```python
from build123d import *

# Parameters (mm, degrees)
SKETCH1_R           = 62.5
SKETCH1_R_2         = 1.75
SKETCH1_R_3         = 19.5
BOSS_EXTRUDE1_DEPTH = 2


with BuildPart() as part:
    # Sketch1 → Boss-Extrude1 (new body)
    with BuildSketch(Plane(origin=(0, 0, 0), x_dir=(1, 0, 0), z_dir=(0, 1, 0))):
        with Locations(Location((0, 0, 0), (0, 0, 270))):
            Circle(SKETCH1_R)
        with Locations(Location((6.153691309, -23.5, 0), (0, 0, 270))):
            Circle(SKETCH1_R_2, mode=Mode.SUBTRACT)
        with Locations(Location((-5.846308691, -23.5, 0), (0, 0, 270))):
            Circle(SKETCH1_R_2, mode=Mode.SUBTRACT)
        with Locations(Location((6.153691309, -56.5, 0), (0, 0, 270))):
            Circle(SKETCH1_R_2, mode=Mode.SUBTRACT)
        with Locations(Location((-5.846308691, -56.5, 0), (0, 0, 270))):
            Circle(SKETCH1_R_2, mode=Mode.SUBTRACT)
        with Locations(Location((-46.007280968, 33.313051845, 0), (0, 0, 270))):
            Circle(SKETCH1_R_2, mode=Mode.SUBTRACT)
        with Locations(Location((-23.428442643, 6.420747, 0), (0, 0, 270))):
            Circle(SKETCH1_R_2, mode=Mode.SUBTRACT)
        with Locations(Location((-17.428442643, 16.813051845, 0), (0, 0, 270))):
            Circle(SKETCH1_R_2, mode=Mode.SUBTRACT)
        with Locations(Location((-52.007280968, 22.920747, 0), (0, 0, 270))):
            Circle(SKETCH1_R_2, mode=Mode.SUBTRACT)
        with Locations(Location((51.853589659, 23.186948155, 0), (0, 0, 270))):
            Circle(SKETCH1_R_2, mode=Mode.SUBTRACT)
        with Locations(Location((17.274751335, 17.079253, 0), (0, 0, 270))):
            Circle(SKETCH1_R_2, mode=Mode.SUBTRACT)
        with Locations(Location((23.274751335, 6.686948155, 0), (0, 0, 270))):
            Circle(SKETCH1_R_2, mode=Mode.SUBTRACT)
        with Locations(Location((45.853589659, 33.579253, 0), (0, 0, 270))):
            Circle(SKETCH1_R_2, mode=Mode.SUBTRACT)
        with Locations(Location((0, 0, 0), (0, 0, 270))):
            Circle(SKETCH1_R_3, mode=Mode.SUBTRACT)
        with Locations(Location((0, 30, 0), (0, 0, 270))):
            Circle(SKETCH1_R_2, mode=Mode.SUBTRACT)
        with Locations(Location((25.980762114, -15, 0), (0, 0, 270))):
            Circle(SKETCH1_R_2, mode=Mode.SUBTRACT)
        with Locations(Location((-25.980762114, -15, 0), (0, 0, 270))):
            Circle(SKETCH1_R_2, mode=Mode.SUBTRACT)
    extrude(amount=BOSS_EXTRUDE1_DEPTH)


solid = part.part
```
CAD build for the part. Positions are in the model's coordinates, mm. Coordinates: 2 decimals unless noted, no trailing zeros. Write each loop counter-clockwise with the first axis right and the second up, starting at its lowest first coordinate (ties: lowest second). Pieces come first, ordered by that corner, then holes. Notation, with made-up numbers: (-7, 63) -> (41, 63) arc R26 cw to (41, 95) -> close; hole circle Ø6 at (0, 2). An arc over 180 degrees is marked (long way). Return JSON: item names as keys, results as strings. Group by question number.
Q1. Flat gauge pins, fed straight in: pin 1 (4.5 mm diameter, centred on x = -17.43, z = -16.81, fed in from +Y); pin 2 (1 mm diameter, centred on y = 0.5, z = 39.5, fed in from +X). Where does each tip first touch, or does it go through?
Q2. Cut at C-C, the plane y = 1.35. State how many separate pieces and enclosed holes the cut face has, then the cut area to 3 significant figures.
Q3. Cut at B-B, the plane z = 0. Give the cut face in (x, y), then the cut area to 3 significant figures.
Q4. Drill centre lines: line 1 (X direction, y = 0.2, z = 55); line 2 (X direction, y = 1.2, z = 0); line 3 (X direction, y = 1.2, z = 23.5). Where is each one in solid material? Low to high.
Q5. Pull direction X, two halves, no side cores. Call faces 1 (the face through (2.75, 0.99, -62.44)), 2 (the face through (15, 2, 13)), 3 (the face through (-25.46, 0.99, 16.67)): released by +X, released by -X, zero draft, split by the parting line, or undercut.
Q6. Cut at A-A, the plane x = 0. Give the cut face in (y, z).
Q7. Cut at D-D, the plane z = 15. Give the cut face in (x, y).
Returned:
{
 "1": {"pin 1": "stops at y = 2", "pin 2": "stops at x = 48.84"},
 "2": {"separate pieces": "1", "enclosed holes": "16", "area": "10,900 mm2"},
 "3": {"outline": "(-62.5, 0) -> (-19.5, 0) -> (-19.5, 2) -> (-62.5, 2) -> close; (19.5, 0) -> (62.5, 0) -> (62.5, 2) -> (19.5, 2) -> close", "area": "172 mm2"},
 "4": {"line 1": "x = -29.69 to -6.75, -4.94 to 5.25, 7.06 to 29.69", "line 2": "x = -62.5 to -19.5, 19.5 to 62.5", "line 3": "x = -57.91 to -7.6, -4.1 to 4.4, 7.9 to 57.91"},
 "5": {"face 1": "split by the parting line", "face 2": "zero draft", "face 3": "undercut"},
 "6": {"outline": "(0, -62.5) -> (2, -62.5) -> (2, -31.75) -> (0, -31.75) -> close; (0, -28.25) -> (2, -28.25) -> (2, -19.5) -> (0, -19.5) -> close; (0, 19.5) -> (2, 19.5) -> (2, 62.5) -> (0, 62.5) -> close"},
 "7": {"outline": "(-60.67, 0) -> (-27.73, 0) -> (-27.73, 2) -> (-60.67, 2) -> close; (-24.23, 0) -> (-12.46, 0) -> (-12.46, 2) -> (-24.23, 2) -> close; (12.46, 0) -> (24.23, 0) -> (24.23, 2) -> (12.46, 2) -> close; (27.73, 0) -> (60.67, 0) -> (60.67, 2) -> (27.73, 2) -> close"}
}
